For this review, use the dimensioned drawing (mm, ordinates from the lowest corner) and the shaded views. Coordinates: 2 decimals unless noted, no trailing zeros. Write each loop counter-clockwise with the first axis right and the second up, starting at its lowest first coordinate (ties: lowest second). Pieces come first, ordered by that corner, then holes. Notation, with made-up numbers: M -3,9.5 L 41,9.5 A22 ccw 41,36.5 Z; hole C 89,-11.75 d4. An arc over 180 degrees is marked long. One line per question, with ' | ' between items.
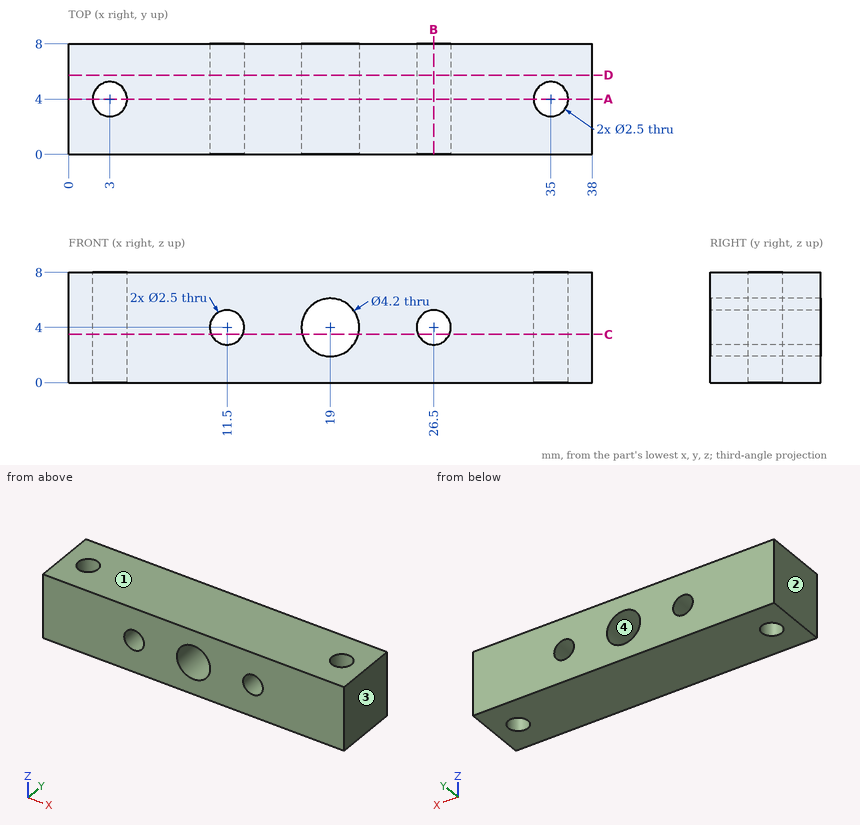
1) To check wall thickness, follow line 1 along X through (y, z) = (5.5, 4.5); line 2 along Y through (x, z) = (35, 3.5). State the ranges of each line that lie inside material, in increasing order. Write a range as [from, to].
Responses:
line 1: [0, 10.35], [12.65, 16.96], [21.04, 25.35], [27.65, 38] | line 2: [0, 2.75], [5.25, 8]
2) The part is to be moulded in two halves that separate along X. For the marked faces 1, 2, 3 and 4, say which applies: +X half, -X half, draft (parallel to the pull), parting line (faces both ways), or undercut.
Responses:
face 1: draft | face 2: -X half | face 3: +X half | face 4: undercut
3) We need section B-B on x = 26.5. State the section outline as (y, z) points, then the cut area to 3 significant figures.
Responses:
outline: M 0,0 L 8,0 L 8,2.75 L 0,2.75 Z; M 0,5.25 L 8,5.25 L 8,8 L 0,8 Z | area: 44.0 mm^2
4) We need section A-A on y = 4. State the section outline as (x, z) points.
Responses:
outline: M 0,0 L 1.75,0 L 1.75,8 L 0,8 Z; M 4.25,0 L 33.75,0 L 33.75,8 L 4.25,8 Z; M 36.25,0 L 38,0 L 38,8 L 36.25,8 Z; hole C 11.5,4 d2.5; hole C 19,4 d4.2; hole C 26.5,4 d2.5
5) We need section C-C on z = 3.5. State the section outline as (x, y) points.
Responses:
outline: M 0,0 L 10.35,0 L 10.35,8 L 0,8 Z; M 12.65,0 L 16.96,0 L 16.96,8 L 12.65,8 Z; M 21.04,0 L 25.35,0 L 25.35,8 L 21.04,8 Z; M 27.65,0 L 38,0 L 38,8 L 27.65,8 Z; hole C 3,4 d2.5; hole C 35,4 d2.5
6) We need section D-D on y = 5.75. State the section outline as (x, z) points.
Responses:
outline: M 0,0 L 38,0 L 38,8 L 0,8 Z; hole C 11.5,4 d2.5; hole C 19,4 d4.2; hole C 26.5,4 d2.5
